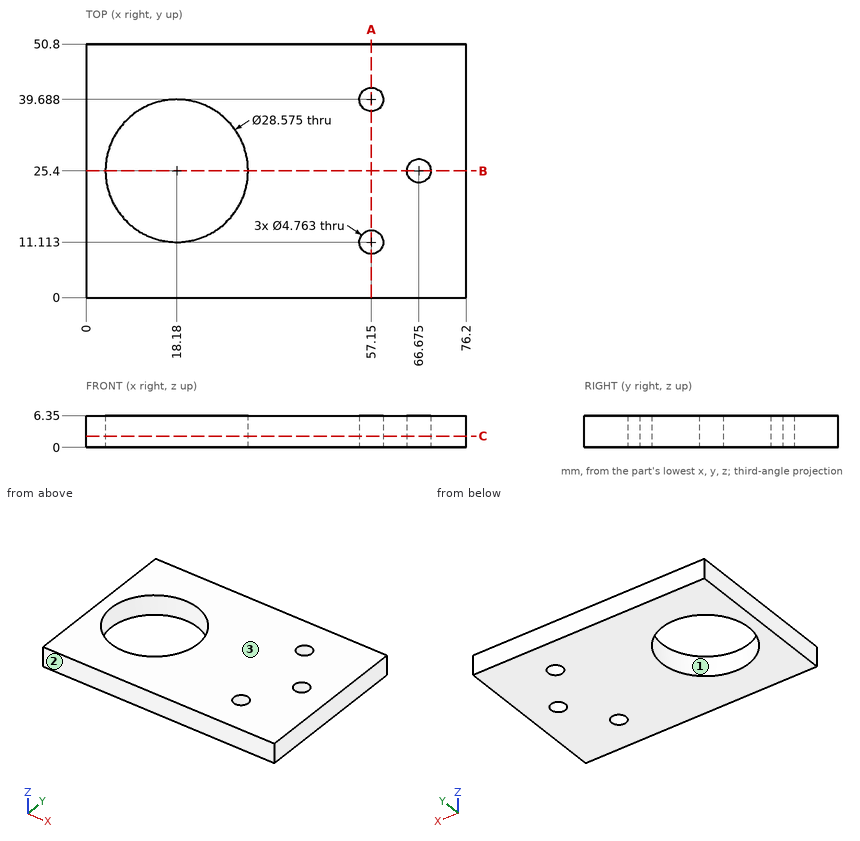
Study the drawing (mm; zero at the part's minimum x, y, z) and answer. Give positions to 0.01 mm unless a question says otherwise; leave off trailing zeros. Write each loop counter-clockwise with the first axis right and the second up, starting at its lowest first coordinate (ties: lowest second). Pieces come first, ordered by that corner, then holes. Notation, with made-up numbers: (24.25, -35) -> (34.25, -35) arc R16 ccw to (34.25, -29) -> close; hole circle Ø5 at (78.25, 64). An arc over 180 degrees is marked (long way). Write item = value, one per line.
Q1. For a pull along Y with two mould halves and no side action, classify the marked faces 1, 2 and 3 as pulls with the +Y half, pulls with the -Y half, needs draft (parallel to the pull), parting line crosses it, or undercut.
Computed values:
face_1 = undercut
face_2 = pulls with the -Y half
face_3 = needs draft
Q2. Section A-A on x = 57.15 is taken. Determine the outline of the cut face in (y, z), and give its area (3 significant figures).
Computed values:
outline = (0, 0) -> (8.73, 0) -> (8.73, 6.35) -> (0, 6.35) -> close; (13.49, 0) -> (37.31, 0) -> (37.31, 6.35) -> (13.49, 6.35) -> close; (42.07, 0) -> (50.8, 0) -> (50.8, 6.35) -> (42.07, 6.35) -> close
area = 262 mm^2
Q3. Section C-C on z = 2.25 is taken. State how many separate pieces and enclosed holes the cut face has, and give its area (3 significant figures).
Computed values:
separate_pieces = 1
enclosed_holes = 4
area = 3,180 mm^2
Q4. Section B-B on y = 25.4 is taken. Determine the outline of the cut face in (x, z).
Computed values:
outline = (0, 0) -> (3.89, 0) -> (3.89, 6.35) -> (0, 6.35) -> close; (32.47, 0) -> (64.29, 0) -> (64.29, 6.35) -> (32.47, 6.35) -> close; (69.06, 0) -> (76.2, 0) -> (76.2, 6.35) -> (69.06, 6.35) -> close
Q5. Consider line 1 along Y through (x, z) = (57.15, 4.5); line 2 along X through (y, z) = (25, 2.5); line 3 along X through (y, z) = (37, 5.5) (1 decimal). Determine where each line is inside the solid, lowest interval first.
Computed values:
line_1 = 0 to 8.73, 13.49 to 37.31, 42.07 to 50.8
line_2 = 0 to 3.9, 32.46 to 64.33, 69.02 to 76.2
line_3 = 0 to 9.8, 26.5 to 76.2
